```python
from build123d import *

# Parameters (mm, degrees)
SKETCH2_R           = 4
BOSS_EXTRUDE2_DEPTH = 9.525
SKETCH3_R           = 2
CUT_EXTRUDE1_DEPTH  = 6.35


with BuildPart() as part:
    # Sketch2 → Boss-Extrude2 (new, symmetric)
    with BuildSketch(Plane(origin=(0, 0, 0), x_dir=(1, 0, 0), z_dir=(0, 1, 0))):
        with Locations(Location((0, 0, 0), (0, 0, 90))):
            Circle(SKETCH2_R)
    extrude(amount=BOSS_EXTRUDE2_DEPTH, both=True)

    # Sketch3 → Cut-Extrude1 (cut)
    with BuildSketch(Plane(origin=(0, 9.525, 0), x_dir=(1, 0, 0), z_dir=(0, 1, 0))):
        with Locations(Location((0, 0, 0), (0, 0, 270))):
            Circle(SKETCH3_R)
    cut_extrude1 = extrude(amount=-CUT_EXTRUDE1_DEPTH, mode=Mode.SUBTRACT)

    # Mirror1: Cut-Extrude1 across plane
    add(cut_extrude1.mirror(Plane.ZX), mode=Mode.SUBTRACT)


solid = part.part
```
The model under review builds one solid part; all positions refer to its coordinate system, in mm. A direction names the side the tool comes from. Round coordinates to 2 decimals unless told otherwise and drop trailing zeros. Order: outer loops, then holes, each group sorted by start corner. A loop starts at its lowest first (then second) coordinate and runs counter-clockwise, first axis right, second up. Notation, with made-up numbers: M 72.5,73 L 104.5,73 A15 cw 104.5,77 Z; hole C 3,-19.75 d7. An arc over 180 degrees is marked long. Use a Markdown table: item, result.
1) Consider section A-A (z = 0). Write out the cut boundary in (x, y) (3 decimals).
Report:
| item | result |
|---|---|
| outline | M -4,-9.525 L -2,-9.525 L -2,-3.175 L 2,-3.175 L 2,-9.525 L 4,-9.525 L 4,9.525 L 2,9.525 L 2,3.175 L -2,3.175 L -2,9.525 L -4,9.525 Z |
2) Consider section B-B (x = 0). Write out the cut boundary in (y, z) (3 decimals).
Report:
| item | result |
|---|---|
| outline | M -9.525,-4 L 9.525,-4 L 9.525,-2 L 3.175,-2 L 3.175,2 L 9.525,2 L 9.525,4 L -9.525,4 L -9.525,2 L -3.175,2 L -3.175,-2 L -9.525,-2 Z |
3) Wall thickness on line 1 along X through (y, z) = (7.25, 0); line 2 along Y through (x, z) = (1.5, -1.25) (3 decimals); line 3 along Z through (x, y) = (0.5, -6.5): over which ranges is each line inside the solid? List them lowest first. Write a range as [from, to].
Report:
| item | result |
|---|---|
| line 1 | [-4, -2], [2, 4] |
| line 2 | [-3.175, 3.175] |
| line 3 | [-3.97, -1.94], [1.94, 3.97] |
4) Draft analysis for pull direction X (two halves, no side actions). For faces 1 (the face through (1, 9.525, 2)), 2 (the face through (3.905, 0.133, 0.867)), 3 (the face through (0, -3.175, 0)), 4 (the face through (-2, -6, 0)), state which applies: released by +X, released by -X, zero draft, split by the parting line, or undercut.
Report:
| item | result |
|---|---|
| face 1 | zero draft |
| face 2 | split by the parting line |
| face 3 | undercut |
| face 4 | undercut |
5) Consider section C-C (y = 5.75). Write out the cut boundary in (x, z).
Report:
| item | result |
|---|---|
| outline | C 0,0 d8; hole C 0,0 d4 |
6) Tool access review of faces 5 (the face through (1, -9.525, 2)), 6 (the face through (0, 3.175, 0)): name each direction out of +Z, -Z, +X, -X, +Y, -Y from which nothing blocks a thin tool from reaching the whole face with its end or side.
Report:
| item | result |
|---|---|
| face 5 | +Z, -Z, +X, -X, -Y |
| face 6 | +Y |
7) Insertion check: pin 1 (3.5 mm diameter, centred on x = 0, z = 0, fed in from +Y) (3 decimals); pin 2 (2 mm diameter, centred on y = -5.5, z = 2, fed in from -X); pin 3 (4 mm diameter, centred on x = 3, y = -5.5, fed in from +Z). Each pin has a flat end and moves straight along its axis. Give the tip position at first contact, or say it passes through.
Report:
| item | result |
|---|---|
| pin 1 | y = 3.175 |
| pin 2 | x = -3.87 |
| pin 3 | z = 3.87 |
